CAD build for the part. Positions are in the model's coordinates, mm. Face numbers are marked on the shaded views. Round coordinates to 2 decimals unless told otherwise and drop trailing zeros. Loops run counter-clockwise (first coordinate to the right, second up) from the corner with the lowest first, then second, coordinate; pieces in that order, holes last.
from build123d import *

# Parameters (mm, degrees)
SKETCH1_W           = 32
SKETCH1_H           = 32
BOSS_EXTRUDE1_DEPTH = 7
LPATTERN2_COUNT     = 2
LPATTERN2_PITCH     = 16


with BuildPart() as part:
    # Sketch1 → Boss-Extrude1 (new body)
    with BuildSketch(Plane(origin=(0, 0, 0), x_dir=(1, 0, 0), z_dir=(0, 1, 0))):
        Rectangle(SKETCH1_W, SKETCH1_H)
    extrude(amount=BOSS_EXTRUDE1_DEPTH)

    # Sketch3 → CSK for M1.6 Countersunk Flat Head Screw1 (revolve, cut)
    with BuildSketch(Plane(origin=(8, 0, 0), x_dir=(0, 0, -1), z_dir=(1, 0, 0))):
        Polygon((0, 0), (0, 7), (3.5, 7), (3.5, 4.999754046), (6.5, 0), align=None)
    csk_for_m1_6_countersunk_flat_head_screw = revolve(axis=Axis((8, -6.35, 0), (0, 1, 0)), mode=Mode.SUBTRACT)

    # LPattern2: CSK for M1.6 Countersunk Flat Head Screw1 ×2
    with Locations(*[(-i * LPATTERN2_PITCH, 0, 0) for i in range(1, LPATTERN2_COUNT)]):
        add(csk_for_m1_6_countersunk_flat_head_screw, mode=Mode.SUBTRACT)


solid = part.part
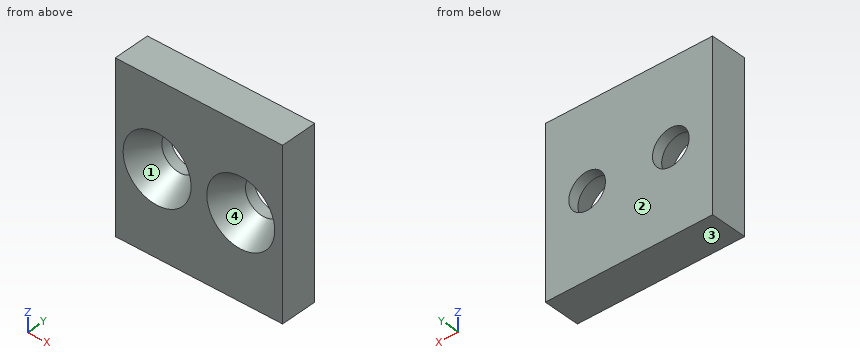
Item 1: Cut at D-D (y = 3). List the corners of the cut face in (x, z), plus the area to 3 significant figures.
Verdict:
outline: (-16, -16) - (16, -16) - (16, 16) - (-16, 16) - close; hole circle Ø9.4 at (-8, 0); hole circle Ø9.4 at (8, 0)
area: 885 mm2
Item 2: Cut at B-B (x = 8). List the corners of the cut face in (y, z).
Verdict:
outline: (0, -16) - (7, -16) - (7, -3.5) - (5, -3.5) - (0, -6.5) - close; (0, 6.5) - (5, 3.5) - (7, 3.5) - (7, 16) - (0, 16) - close
Item 3: Wall check: L1, parallel to X at y = 6.4, z = 0; L2, parallel to Z at x = 8, y = 6.05; L3, parallel to X at y = 1, z = 4. Give the ranges that are in metal, low to high.
Verdict:
L1: x = -16 to -11.5, -4.5 to 4.5, 11.5 to 16
L2: z = -16 to -3.5, 3.5 to 16
L3: x = -16 to -12.34, -3.66 to 3.66, 12.34 to 16
Item 4: Cut at C-C (y = 6.25). List the corners of the cut face in (x, z).
Verdict:
outline: (-16, -16) - (16, -16) - (16, 16) - (-16, 16) - close; hole circle Ø7 at (-8, 0); hole circle Ø7 at (8, 0)
Item 5: Mould opens along Z. For the marked faces 1, 2, 3 and 4 say: released by +Z, released by -Z, zero draft, split by the parting line, or undercut.
Verdict:
face 1: undercut
face 2: zero draft
face 3: released by -Z
face 4: undercut
Item 6: Flat gauge pins, fed straight in: P1, Ø5.5, axis at x = -8, z = 0, coming from the -Y side; P2, Ø5, axis at x = 11, z = 1.5, coming from the -Y side; P3, Ø11, axis at x = 8, z = 0, coming from the -Y side; P4, Ø2, axis at x = -8.5, z = -3, coming from the -Y side. Where does each tip first touch, or does it go through?
Verdict:
P1: passes through
P2: stops at y = 1.08
P3: stops at y = 1.67
P4: stops at y = 4.1
Item 7: Cut at A-A (z = 0). List the corners of the cut face in (x, y), plus the area to 3 significant figures.
Verdict:
outline: (-16, 0) - (-14.5, 0) - (-11.5, 5) - (-11.5, 7) - (-16, 7) - close; (-4.5, 5) - (-1.5, 0) - (1.5, 0) - (4.5, 5) - (4.5, 7) - (-4.5, 7) - close; (11.5, 5) - (14.5, 0) - (16, 0) - (16, 7) - (11.5, 7) - close
area: 96.0 mm2
